Check sheet for the modelled part. Datum: model origin and axes. Units: mm. A direction names the side the tool comes from. Coordinates: 2 decimals unless noted, no trailing zeros. Order: outer loops, then holes, each group sorted by start corner. A loop starts at its lowest first (then second) coordinate and runs counter-clockwise, first axis right, second up.
from build123d import *

# Parameters (mm, degrees)
ESBO_O1_W                = 100
ESBO_O1_H                = 70
RESSALTO_EXTRUS_O1_DEPTH = 50
ESBO_O3_W                = 45
ESBO_O3_H                = 30
CORTE_EXTRUS_O1_DEPTH    = 118.153745139
ESBO_O4_W                = 45
ESBO_O4_H                = 60
CORTE_EXTRUS_O2_DEPTH    = 100.498743711
ESBO_O5_R                = 15
CORTE_EXTRUS_O3_DEPTH    = 79.89866919
ESBO_O6_R                = 4
CORTE_EXTRUS_O4_DEPTH    = 79.89866919
ESBO_O6_3_R              = 4
CORTE_EXTRUS_O5_DEPTH    = 50
ESBO_O6_4_R              = 4
CORTE_EXTRUS_O6_DEPTH    = 50
ESBO_O6_5_R              = 4
CORTE_EXTRUS_O7_DEPTH    = 50
ESBO_O6_6_R              = 4
CORTE_EXTRUS_O8_DEPTH    = 50
ESBO_O6_7_R              = 4
CORTE_EXTRUS_O9_DEPTH    = 50
ESBO_O6_8_R              = 4
CORTE_EXTRUS_O10_DEPTH   = 50
ESBO_O8_R                = 4
CORTE_EXTRUS_O11_DEPTH   = 50
ESBO_O9_R                = 4
CORTE_EXTRUS_O12_DEPTH   = 118.153745139
ESBO_O10_R               = 4
CORTE_EXTRUS_O13_DEPTH   = 118.153745139
FILETE2_R                = 10
FILETE3_R                = 10
FILETE4_R                = 10
FILETE5_R                = 10


with BuildPart() as part:
    # Esboço1 → Ressalto-extrusão1 (new body)
    with BuildSketch(Plane(origin=(0, 0, 0), x_dir=(0, 0, -1), z_dir=(1, 0, 0))):
        Rectangle(ESBO_O1_W, ESBO_O1_H)
    extrude(amount=RESSALTO_EXTRUS_O1_DEPTH)

    # Esboço3 → Corte-extrusão1 (cut, through all)
    with BuildSketch(Plane.XY.offset(50)):
        with Locations((27.5, 0)):
            Rectangle(ESBO_O3_W, ESBO_O3_H)
    extrude(amount=-CORTE_EXTRUS_O1_DEPTH, mode=Mode.SUBTRACT)

    # Esboço4 → Corte-extrusão2 (cut, through all)
    with BuildSketch(Plane(origin=(0, -35, 0), x_dir=(-1, 0, 0), z_dir=(0, -1, 0))):
        with Locations((-27.5, 0)):
            Rectangle(ESBO_O4_W, ESBO_O4_H)
    extrude(amount=-CORTE_EXTRUS_O2_DEPTH, mode=Mode.SUBTRACT)

    # Esboço5 → Corte-extrusão3 (cut, through all)
    with BuildSketch(Plane.ZY):
        Circle(ESBO_O5_R)
    extrude(amount=-CORTE_EXTRUS_O3_DEPTH, mode=Mode.SUBTRACT)

    # Esboço6 → Corte-extrusão4 (cut, through all)
    with BuildSketch(Plane.ZY):
        with Locations((-25, 0)):
            Circle(ESBO_O6_R)
    extrude(amount=-CORTE_EXTRUS_O4_DEPTH, mode=Mode.SUBTRACT)

    # Esboço6<3> → Corte-extrusão5 (cut)
    with BuildSketch(Plane.ZY):
        with Locations((-17.67766953, -17.67766953)):
            Circle(ESBO_O6_3_R)
    extrude(amount=-CORTE_EXTRUS_O5_DEPTH, mode=Mode.SUBTRACT)

    # Esboço6<4> → Corte-extrusão6 (cut)
    with BuildSketch(Plane.ZY):
        with Locations((0, -25)):
            Circle(ESBO_O6_4_R)
    extrude(amount=-CORTE_EXTRUS_O6_DEPTH, mode=Mode.SUBTRACT)

    # Esboço6<5> → Corte-extrusão7 (cut)
    with BuildSketch(Plane.ZY):
        with Locations((17.67766953, -17.67766953)):
            Circle(ESBO_O6_5_R)
    extrude(amount=-CORTE_EXTRUS_O7_DEPTH, mode=Mode.SUBTRACT)

    # Esboço6<6> → Corte-extrusão8 (cut)
    with BuildSketch(Plane.ZY):
        with Locations((25, 0)):
            Circle(ESBO_O6_6_R)
    extrude(amount=-CORTE_EXTRUS_O8_DEPTH, mode=Mode.SUBTRACT)

    # Esboço6<7> → Corte-extrusão9 (cut)
    with BuildSketch(Plane.ZY):
        with Locations((17.67766953, 17.67766953)):
            Circle(ESBO_O6_7_R)
    extrude(amount=-CORTE_EXTRUS_O9_DEPTH, mode=Mode.SUBTRACT)

    # Esboço6<8> → Corte-extrusão10 (cut)
    with BuildSketch(Plane.ZY):
        with Locations((0, 25)):
            Circle(ESBO_O6_8_R)
    extrude(amount=-CORTE_EXTRUS_O10_DEPTH, mode=Mode.SUBTRACT)

    # Esboço8 → Corte-extrusão11 (cut)
    with BuildSketch(Plane.ZY):
        with Locations((-18.018451128, 17.56107414)):
            Circle(ESBO_O8_R)
    extrude(amount=-CORTE_EXTRUS_O11_DEPTH, mode=Mode.SUBTRACT)

    # Esboço9 → Corte-extrusão12 (cut, through all)
    with BuildSketch(Plane.XY.offset(50)):
        with Locations((25, -25)):
            Circle(ESBO_O9_R)
    extrude(amount=-CORTE_EXTRUS_O12_DEPTH, mode=Mode.SUBTRACT)

    # Esboço10 → Corte-extrusão13 (cut, through all)
    with BuildSketch(Plane.XY.offset(50)):
        with Locations((25, 25)):
            Circle(ESBO_O10_R)
    extrude(amount=-CORTE_EXTRUS_O13_DEPTH, mode=Mode.SUBTRACT)

    # Filete2
    # the kernel refuses this fillet: 10 mm, written as the material it takes off along each edge
    with BuildSketch(Plane(origin=(-25, -35, 50), x_dir=(0, 1, 0), z_dir=(1, 0, 0))) as filete2_piece_1:
        with BuildLine():
            CenterArc((FILETE2_R, -FILETE2_R), FILETE2_R, 90, 90)
            Line((0, -FILETE2_R), (0, 0))
            Line((0, 0), (FILETE2_R, 0))
        make_face()
    extrude(amount=100, mode=Mode.SUBTRACT)

    # Filete3
    # the kernel refuses this fillet: 10 mm, written as the material it takes off along each edge
    with BuildSketch(Plane(origin=(-25, 35, 50), x_dir=(0, 0, -1), z_dir=(1, 0, 0))) as filete3_piece_1:
        with BuildLine():
            CenterArc((FILETE3_R, -FILETE3_R), FILETE3_R, 90, 90)
            Line((0, -FILETE3_R), (0, 0))
            Line((0, 0), (FILETE3_R, 0))
        make_face()
    extrude(amount=100, mode=Mode.SUBTRACT)

    # Filete4
    # the kernel refuses this fillet: 10 mm, written as the material it takes off along each edge
    with BuildSketch(Plane(origin=(-25, 35, -50), x_dir=(0, 0, 1), z_dir=(1, 0, 0))) as filete4_piece_1:
        with BuildLine():
            CenterArc((FILETE4_R, FILETE4_R), FILETE4_R, 180, 90)
            Line((0, FILETE4_R), (0, 0))
            Line((0, 0), (FILETE4_R, 0))
        make_face()
    extrude(amount=100, mode=Mode.SUBTRACT)

    # Filete5
    # the kernel refuses this fillet: 10 mm, written as the material it takes off along each edge
    with BuildSketch(Plane(origin=(-25, -35, -50), x_dir=(0, 0, 1), z_dir=(1, 0, 0))) as filete5_piece_1:
        with BuildLine():
            CenterArc((FILETE5_R, -FILETE5_R), FILETE5_R, 90, 90)
            Line((0, -FILETE5_R), (0, 0))
            Line((0, 0), (FILETE5_R, 0))
        make_face()
    extrude(amount=100, mode=Mode.SUBTRACT)


solid = part.part
(1) Cross-section at A-A (x = 45). Enter the section's corners in (y, z), and give its area (3 significant figures).
Filled in:
outline: (-35, -40) arc R10 ccw to (-25, -50) - (-15, -50) - (-15, -30) - (-35, -30) - close; (-35, 30) - (-15, 30) - (-15, 50) - (-25, 50) arc R10 ccw to (-35, 40) - close; (15, -50) - (25, -50) arc R10 ccw to (35, -40) - (35, -30) - (15, -30) - close; (15, 30) - (35, 30) - (35, 40) arc R10 ccw to (25, 50) - (15, 50) - close
area: 1,510 mm2
(2) Cross-section at B-B (z = 0). Enter the section's corners in (x, y), and give its area (3 significant figures).
Filled in:
outline: (0, -35) - (5, -35) - (5, -29) - (0, -29) - close; (0, -21) - (5, -21) - (5, -15) - (0, -15) - close; (0, 15) - (5, 15) - (5, 21) - (0, 21) - close; (0, 29) - (5, 29) - (5, 35) - (0, 35) - close
area: 120 mm2
(3) Release check for a two-part mould opening along X. For faces 3 (the flat face through (0, 16, 1)), 4 (the cylindrical face through (2.465, 0.66, -14.985)), 5 (the cylindrical face through (24.479, 28.966, -39.86)), 6 (the cylindrical face through (24.479, 28.966, 40.14)) record: +X half, -X half, draft (parallel to the pull), parting line (faces both ways), or undercut.
Filled in:
face 3: -X half
face 4: draft
face 5: undercut
face 6: undercut
(4) Cross-section at C-C (y = 0). Enter the section's corners in (x, z), and give its area (3 significant figures).
Filled in:
outline: (0, -50) - (5, -50) - (5, -29) - (0, -29) - close; (0, -21) - (5, -21) - (5, -15) - (0, -15) - close; (0, 15) - (5, 15) - (5, 21) - (0, 21) - close; (0, 29) - (5, 29) - (5, 50) - (0, 50) - close
area: 270 mm2
(5) Thickness scan on probe 1 along Y at (x, z) = (25, -33.5); probe 2 along Z at (x, y) = (37, -15.5); probe 3 along Y at (x, z) = (25, 44.5). Record the ranges inside material, lowest first.
Filled in:
probe 1: y = -35 to -29, -21 to -15, 15 to 21, 29 to 35
probe 2: z = -50 to -30, 30 to 50
probe 3: y = -33.93 to -29, -21 to -15, 15 to 21, 29 to 33.93
(6) Tool access check on faces 1 (the flat face through (27, -15, 40)), 2 (the cylindrical face through (24.65, 32.15, 46.99)). Record the directions out of +Z, -Z, +X, -X, +Y, -Y that give a thin tool (end or side, any length) a straight path to the whole face; none if there is none.
Filled in:
face 1: +Z, -Z, +X
face 2: +Z, +X, -X, +Y
(7) Cross-section at D-D (z = 34.5). Enter the section's corners in (x, y), and give its area (3 significant figures).
Filled in:
outline: (0, -35) - (50, -35) - (50, -15) - (5, -15) - (5, 15) - (50, 15) - (50, 35) - (0, 35) - close; hole circle Ø8 at (25, -25); hole circle Ø8 at (25, 25)
area: 2,050 mm2
(8) Go/stop test with a flat-tipped pin: P1, Ø6, axis at y = -5, z = 13.5, coming from the +X side. Record where the tip stops, or that it passes through.
Filled in:
P1: stops at x = 5
